```python
from build123d import *

# Parameters (mm, degrees)
F0_R        = 24.2537643176
F1_DEPTH    = 5
F2_W        = 45.0000017881
F2_H        = 18.5869578272
F3_DEPTH    = 25
F4_W        = 45.0000017881
F4_H        = 5.7842824608
F5_DEPTH    = 5
F6_DEPTH    = 5
F6_TAPER    = -3
F7_DEPTH    = 5
F7_TAPER    = -3
F8_R        = 5
F9_T4_DEPTH = 43.1102228968
F9_S5_R     = 24.2537643176
F9_T6_DEPTH = 23


# Not quite as in the source:
# - a fillet or chamfer that OpenCascade refuses, or shapes differently, is made with other operations: its cross-section is extruded or revolved along the edge and cut away or added


with BuildPart() as f1:
    # F0 (on Top) → F1 (new body)
    with BuildSketch(Plane.XY):
        Circle(F0_R)
    extrude(amount=F1_DEPTH)

    # F2 (on Top) → F3 (join)
    with BuildSketch(Plane.XY):
        Rectangle(F2_W, F2_H)
    extrude(amount=F3_DEPTH)

    # F4 (on face) → F5 (join)
    with BuildSketch(Plane.XY.offset(25)):
        with Locations((0, 0.3060454037)):
            Rectangle(F4_W, F4_H)
    extrude(amount=-F5_DEPTH)

    # F4 (on face) → F6 (join)
    with BuildSketch(Plane.XY.offset(25)):
        with Locations((0, 0.3060454037)):
            Rectangle(F4_W, F4_H)
    extrude(amount=-F6_DEPTH, taper=F6_TAPER)

    # F4 (on face) → F7 (cut)
    with BuildSketch(Plane.XY.offset(25)):
        with Locations((0, 0.3060454037)):
            Rectangle(F4_W, F4_H)
    extrude(amount=-F7_DEPTH, taper=F7_TAPER, mode=Mode.SUBTRACT)

    # F8
    f8_edges = [f1.edges().sort_by_distance(p)[0] for p in [
        (0, -9.293479, 5),
    ]]
    fillet(f8_edges, radius=F8_R)

    # F9: fillet of radius 5 on 1 edges, made by hand


with BuildPart() as f9_tool2:
    # F9_s3 → F9_t4 (new body)
    with BuildSketch(Plane.XZ.offset(21.5551114484)):
        with BuildLine():
            ThreePointArc((-22.5000008941, 10), (-23.9644669881, 6.4644660941), (-27.5000008941, 5))
            Line((-27.5000008941, 5), (-22.5000008941, 5))
            Line((-22.5000008941, 5), (-22.5000008941, 10))
        make_face()
    extrude(amount=-F9_T4_DEPTH)

    # F9_s5 → F9_t6 (intersect, symmetric)
    with BuildSketch(Plane.XY.offset(7.5)):
        Circle(F9_S5_R)
    extrude(amount=F9_T6_DEPTH, both=True, mode=Mode.INTERSECT)


with BuildPart() as f1_1:
    add(f1.part)

    # F9_t1: union F9_tool2
    add(f9_tool2.part)


solid = f1_1.part
```
The listing builds one solid part. Answer for the finished solid, in the listing's coordinates (mm). A direction names the side the tool comes from. Give positions to 0.01 mm unless a question says otherwise; leave off trailing zeros. Loops run counter-clockwise (first coordinate to the right, second up) from the corner with the lowest first, then second, coordinate; pieces in that order, holes last. Notation, with made-up numbers: (16, -26) - (41, -26) arc R16 ccw to (41, -16) - close; hole circle Ø9 at (71.5, 24). An arc over 180 degrees is marked (long way). Return JSON: item names as keys, results as strings. Group by question number.
1. Determine the mould class of faces 1 (the flat face through (0, 9.293, 15)), 2 (the flat face through (0, 0, 20)), 3 (the cylindrical face through (-24.253, 0.13, 3.959)), 4 (the flat face through (22.5, 0, 15)) for opening direction Y: pulls with the +Y half, pulls with the -Y half, needs draft (parallel to the pull), parting line crosses it, or undercut.
2. Given pin 1 Ø6 at (x, z) = (-17.5, 4.5) entering from +Y; pin 2 Ø12 at (y, z) = (-15, 11) entering from +X; pin 3 Ø8 at (x, z) = (11, 5) entering from -Y, each flat-ended and moving along its own axis, determine where each tip first touches the part or whether it passes through.
3. Find section D-D (y = -20). Write down the section's boundary in (x, z).
4. Which of the six approach directions +Z, -Z, +X, -X, +Y, -Y give full straight-line access (tool end or side, diameter ignored) to faces 5 (the flat face through (0, 15, 5)), 6 (the flat face through (0, -18, 5)), 7 (the flat face through (23, 0, 5))?
5. Straight lines are drawn through the part: line 1 (Z direction, x = 14, y = 0); line 2 (Z direction, x = 0, y = -18.5); line 3 (Y direction, x = 1, z = 15.25). For each, find the intervals that lie inside material, in ascending order. Write a range as [from, to].
6. Find section A-A (z = 4). Write down the section's boundary in (x, y).
7. Find section C-C (z = 9.25). Write down the section's boundary in (x, y), then the cut area to 3 significant figures.
8. Find section B-B (y = -5). Write down the section's boundary in (x, z), then the cut area to 3 significant figures.
Verdict:
{
 "1": {"face 1": "pulls with the +Y half", "face 2": "undercut", "face 3": "parting line crosses it", "face 4": "needs draft"},
 "2": {"pin 1": "stops at y = 19.44", "pin 2": "stops at x = 22.5", "pin 3": "stops at y = -23.22"},
 "3": {"outline": "(-13.72, 0) - (13.72, 0) - (13.72, 5) - (-13.72, 5) - close"},
 "4": {"face 5": "+Z, +X, -X, +Y", "face 6": "+Z, +X, -X, -Y", "face 7": "+Z, +X, +Y, -Y"},
 "5": {"line 1": "z = [0, 20]", "line 2": "z = [0, 5]", "line 3": "y = [-9.29, 9.29]"},
 "6": {"outline": "(-22.5, -9.29) - (-22.4, -9.29) arc R24.25 ccw to (22.4, -9.29) - (22.5, -9.29) - (22.5, -9.06) arc R24.25 ccw to (22.5, 9.06) - (22.5, 9.29) - (22.4, 9.29) arc R24.25 ccw to (-22.4, 9.29) - (-22.5, 9.29) - (-22.5, 9.06) arc R24.25 ccw to (-22.5, -9.06) - close"},
 "7": {"outline": "(-22.56, -8.91) arc R24.25 ccw to (-22.5, -9.06) - (-22.5, -9.29) - (-22.4, -9.29) arc R24.25 ccw to (-22.38, -9.35) - (22.38, -9.35) arc R24.25 ccw to (22.4, -9.29) - (22.5, -9.29) - (22.5, 9.29) - (-22.5, 9.29) - (-22.5, 9.06) arc R24.25 ccw to (-22.56, 8.91) - close", "area": "840 mm^2"},
 "8": {"outline": "(-23.73, 0) - (23.73, 0) - (23.73, 5) - (22.5, 5) - (22.5, 25) - (-22.5, 25) - (-22.5, 10) arc R5 cw to (-23.73, 6.71) - close", "area": "1,140 mm^2"}
}
